For this review, take the finished solid that the model builds, in its own axes (mm). Face numbers are marked on the shaded views. A direction names the side the tool comes from. Coordinates: 2 decimals unless noted, no trailing zeros. Write each loop counter-clockwise with the first axis right and the second up, starting at its lowest first coordinate (ties: lowest second). Pieces come first, ordered by that corner, then holes.
```python
from build123d import *

# Parameters (mm, degrees)
BOSS_EXTRUDE1_DEPTH = 30
SKETCH2_R           = 0.7493
BOSS_EXTRUDE2_DEPTH = 38.1
SKETCH3_R           = 0.254
BOSS_EXTRUDE3_DEPTH = 3.81
SKETCH5_R           = 0.254
BOSS_EXTRUDE4_DEPTH = 3.81
BOSS_EXTRUDE6_DEPTH = 11.43


with BuildPart() as part:
    # Sketch1 → Boss-Extrude1 (new, symmetric)
    with BuildSketch(Plane(origin=(0, 0, 0), x_dir=(0, 0, -1), z_dir=(1, 0, 0))):
        with BuildLine():
            Line((-25, 2.9), (25, 2.9))
            ThreePointArc((25, 2.9), (27.9, 0), (25, -2.9))
            Line((25, -2.9), (-25, -2.9))
            ThreePointArc((-25, -2.9), (-27.9, 0), (-25, 2.9))
        make_face()
    extrude(amount=BOSS_EXTRUDE1_DEPTH, both=True)

    # Sketch2 → Boss-Extrude2 (add)
    with BuildSketch(Plane(origin=(30, 0, 0), x_dir=(0, 0, -1), z_dir=(1, 0, 0))):
        with Locations(Location((-6.35, 0, 0), (0, 0, 180))):
            Circle(SKETCH2_R)
        with Locations(Location((6.35, 0, 0), (0, 0, 180))):
            Circle(SKETCH2_R)
    extrude(amount=BOSS_EXTRUDE2_DEPTH)

    # Sketch3 → Boss-Extrude3 (add)
    with BuildSketch(Plane(origin=(68.1, 0, 0), x_dir=(0, 0, -1), z_dir=(1, 0, 0))):
        with Locations((-6.35, 0)):
            Circle(SKETCH3_R)
    extrude(amount=BOSS_EXTRUDE3_DEPTH)

    # Sketch5 → Boss-Extrude4 (add)
    with BuildSketch(Plane(origin=(68.1, 0, 0), x_dir=(0, 0, -1), z_dir=(1, 0, 0))):
        with Locations((6.35, 0)):
            Circle(SKETCH5_R)
    extrude(amount=BOSS_EXTRUDE4_DEPTH)

    # Sketch6 → Boss-Extrude6 (add)
    with BuildSketch(Plane(origin=(30, 0, 0), x_dir=(0, 0, -1), z_dir=(1, 0, 0))):
        with BuildLine():
            Line((26.035, -3.175), (-26.035, -3.175))
            ThreePointArc((-26.035, -3.175), (-29.21, 0), (-26.035, 3.175))
            Line((-26.035, 3.175), (26.035, 3.175))
            ThreePointArc((26.035, 3.175), (29.21, 0), (26.035, -3.175))
        make_face()
    extrude(amount=-BOSS_EXTRUDE6_DEPTH)


solid = part.part
```
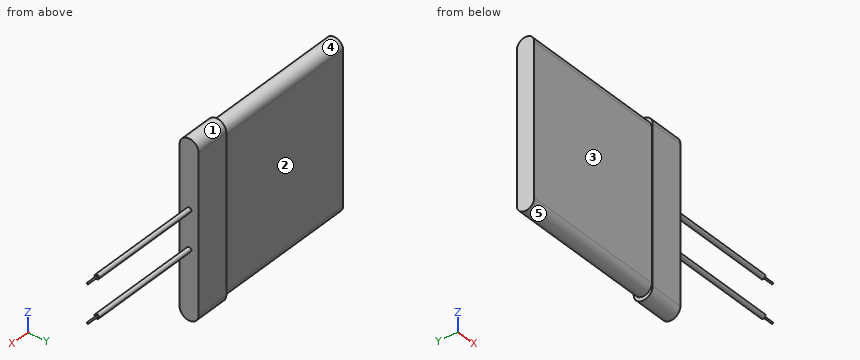
Q1. Add section A-A (z = 0.5). State the section outline as (x, y) points (3 decimals).
Ans:
outline: (-30, -2.9) - (18.57, -2.9) - (18.57, -3.175) - (30, -3.175) - (30, 3.175) - (18.57, 3.175) - (18.57, 2.9) - (-30, 2.9) - close
Q2. Tool access review of the marked faces 1, 2, 3, 4 and 5: name each direction out of +Z, -Z, +X, -X, +Y, -Y from which nothing blocks a thin tool from reaching the whole face with its end or side.
Ans:
face 1: +Z, +X, -X
face 2: +Z, -Z, -X, +Y
face 3: +Z, -Z, -X, -Y
face 4: +Z, -X
face 5: -Z, -X
Q3. For probe 1 along X at (y, z) = (-2.25, 14.5); probe 2 along Z at (x, y) = (55.5, -0.25); probe 3 along Z at (x, y) = (13.5, 0), list the stretches that pass through material, from the lowest coordinate up.
Ans:
probe 1: x = -30 to 30
probe 2: z = -7.06 to -5.64, 5.64 to 7.06
probe 3: z = -27.9 to 27.9
Q4. Clearance check with flat-ended pins moving along their axes: pin 1 Ø14.5 at (x, z) = (-2.5, 10) entering from -Y; pin 2 Ø24.5 at (x, z) = (5, -7) entering from +Y; pin 3 Ø2 at (y, z) = (1.5, 3) entering from +X. State where each tip first meets the part, or that it passes through.
Ans:
pin 1: stops at y = -2.9
pin 2: stops at y = 2.9
pin 3: stops at x = 30
Q5. Add section B-B (x = 31). State the section outline as (y, z) points.
Ans:
outline: circle Ø1.5 at (0, -6.35); circle Ø1.5 at (0, 6.35)
